from build123d import *

# Parameters (mm, degrees)
SKETCH1_W           = 57.16
SKETCH1_H           = 37.39
SKETCH1_W_2         = 40.16
SKETCH1_H_2         = 20.39
BOSS_EXTRUDE1_DEPTH = 5
SKETCH2_W           = 57.16
SKETCH2_H           = 37.39
SKETCH2_W_2         = 40.16
SKETCH2_H_2         = 20.39
BOSS_EXTRUDE2_DEPTH = 28.1
SKETCH3_W           = 48.66
SKETCH3_H           = 8.5
CUT_EXTRUDE1_DEPTH  = 28.1
CUT_EXTRUDE2_REACH  = 63.749
SKETCH5_W           = 16.39
SKETCH5_H           = 10
FILLET1_R           = 4
SKETCH6_R           = 0.95
CUT_EXTRUDE3_DEPTH  = 12
CUT_EXTRUDE4_REACH  = 63.749
SKETCH8_W           = 8.5
SKETCH8_H           = 8.5
BOSS_EXTRUDE3_DEPTH = 14.1
BOSS_EXTRUDE4_REACH = 46.226
SKETCH9_W           = 8.5
SKETCH9_H           = 24.86117923


with BuildPart() as part:
    # Sketch1 → Boss-Extrude1 (new body)
    # profile 1 of 2: a face of its own
    with BuildSketch(Plane(origin=(0, 0, 0), x_dir=(1, 0, 0), z_dir=(0, 1, 0))):
        Rectangle(SKETCH1_W, SKETCH1_H)
        Rectangle(SKETCH1_W_2, SKETCH1_H_2, mode=Mode.SUBTRACT)
    # profile 2 of 2: a face of its own
    with BuildSketch(Plane(origin=(0, 0, 0), x_dir=(1, 0, 0), z_dir=(0, 1, 0))):
        Rectangle(SKETCH1_W_2, SKETCH1_H_2)
    extrude(amount=BOSS_EXTRUDE1_DEPTH)

    # Sketch2 → Boss-Extrude2 (add)
    with BuildSketch(Plane(origin=(0, 5, 0), x_dir=(1, 0, 0), z_dir=(0, 1, 0))):
        Rectangle(SKETCH2_W, SKETCH2_H)
        Rectangle(SKETCH2_W_2, SKETCH2_H_2, mode=Mode.SUBTRACT)
    extrude(amount=BOSS_EXTRUDE2_DEPTH)

    # Sketch3 → Cut-Extrude1 (cut)
    with BuildSketch(Plane(origin=(0, 33.1, 0), x_dir=(1, 0, 0), z_dir=(0, 1, 0))):
        with Locations((-4.25, -14.445)):
            Rectangle(SKETCH3_W, SKETCH3_H)
    extrude(amount=-CUT_EXTRUDE1_DEPTH, mode=Mode.SUBTRACT)

    # Sketch5 → Cut-Extrude2 (cut, up to next)
    with BuildSketch(Plane(origin=(-20.08, 0, 0), x_dir=(0, 0, -1), z_dir=(1, 0, 0)), mode=Mode.PRIVATE) as cut_extrude2_sk1:
        with Locations((-2, 10)):
            Rectangle(SKETCH5_W, SKETCH5_H)
    cut_extrude2_tool1 = extrude(cut_extrude2_sk1.sketch, amount=-CUT_EXTRUDE2_REACH, mode=Mode.PRIVATE) & part.part
    add(cut_extrude2_tool1.solids().sort_by_distance((-20.08, 10, 2))[0], mode=Mode.SUBTRACT)

    # Fillet1
    fillet1_edges = [part.edges().sort_by_distance(p)[0] for p in [
        (-24.33, 15, 10.195),
    ]]
    fillet(fillet1_edges, radius=FILLET1_R)

    # Sketch6 → Cut-Extrude3 (cut)
    with BuildSketch(Plane(origin=(0, 33.1, 0), x_dir=(1, 0, 0), z_dir=(0, 1, 0))):
        with Locations(Location((-24.35, -4.95, 0), (0, 0, 270))):
            Circle(SKETCH6_R)
        with Locations(Location((-24.35, 4.95, 0), (0, 0, 90))):
            Circle(SKETCH6_R)
        with Locations(Location((24.35, 4.95, 0), (0, 0, 270))):
            Circle(SKETCH6_R)
        with Locations(Location((24.35, -4.95, 0), (0, 0, 90))):
            Circle(SKETCH6_R)
    extrude(amount=-CUT_EXTRUDE3_DEPTH, mode=Mode.SUBTRACT)

    # Sketch7 → Cut-Extrude4 (cut, up to next)
    with BuildSketch(Plane.ZY.offset(-20.08), mode=Mode.PRIVATE) as cut_extrude4_sk1:
        with BuildLine():
            Line((10.195, 33.1), (10.195, 19))
            ThreePointArc((10.195, 19), (9.023427125, 16.171572875), (6.195, 15))
            Line((6.195, 15), (-6.195, 15))
            Line((-6.195, 15), (-6.195, 5))
            Line((-6.195, 5), (18.695, 5))
            Line((18.695, 5), (18.695, 33.1))
            Line((18.695, 33.1), (10.195, 33.1))
        make_face()
    cut_extrude4_tool1 = extrude(cut_extrude4_sk1.sketch, amount=-CUT_EXTRUDE4_REACH, mode=Mode.PRIVATE) & part.part
    add(cut_extrude4_tool1.solids().sort_by_distance((20.08, 15.371532, 9.379812))[0], mode=Mode.SUBTRACT)

    # Sketch8 → Boss-Extrude3 (add)
    with BuildSketch(Plane(origin=(0, 33.1, 0), x_dir=(1, 0, 0), z_dir=(0, 1, 0))):
        with Locations((-24.33, -14.445)):
            Rectangle(SKETCH8_W, SKETCH8_H)
    extrude(amount=-BOSS_EXTRUDE3_DEPTH)

    # Sketch9 → Boss-Extrude4 (add, up to next)
    with BuildSketch(Plane(origin=(0, 5, 0), x_dir=(1, 0, 0), z_dir=(0, 1, 0)), mode=Mode.PRIVATE) as boss_extrude4_sk1:
        with Locations((-24.33, -6.235589615)):
            Rectangle(SKETCH9_W, SKETCH9_H)
    boss_extrude4_tool1 = extrude(boss_extrude4_sk1.sketch, amount=BOSS_EXTRUDE4_REACH, mode=Mode.PRIVATE) - part.part
    add(boss_extrude4_tool1.solids().sort_by_distance((-24.33, 5, 6.23559))[0])


solid = part.part
For this review, take the finished solid that the model builds, in its own axes (mm). A direction names the side the tool comes from. Round coordinates to 2 decimals unless told otherwise and drop trailing zeros. Loops run counter-clockwise (first coordinate to the right, second up) from the corner with the lowest first, then second, coordinate; pieces in that order, holes last. Notation, with made-up numbers: (-27.5, 22.25) - (12.5, 22.25) arc R31 cw to (12.5, 52.25) - close; hole circle Ø3 at (86, -11.75). An arc over 180 degrees is marked (long way). One line per item, written item: value. Start each with the question number.
Item 1: Clearance check with flat-ended pins moving along their axes: pin 1 Ø8.5 at (x, y) = (6.5, 21.5) entering from +Z (3 decimals); pin 2 Ø7 at (x, y) = (23, 29) entering from +Z (3 decimals); pin 3 Ø8.5 at (x, z) = (-11, 6.5) entering from +Y. State where each tip first meets the part, or that it passes through.
Item 2: For faces 1 (the flat face through (-20.08, 19, 4)), 2 (the flat face through (24, 26, 10.195)), 3 (the flat face through (24, 10, -6.195)), 4 (the flat face through (-24, 21.1, 5)), list the 3-axis set-ups (+Z, -Z, +X, -X, +Y, -Y) from which the entire face can be reached by the end or side of a thin tool; tool diameter is ignored.
Item 3: For L1, parallel to X at y = 26.25, z = -4.95; L2, parallel to X at y = 16.5, z = 7.5; L3, parallel to Y at x = 14.5, z = 16, list the stretches that pass through material, from the lowest coordinate up.
Item 4: The part is to be moulded in two halves that separate along Y. For faces 5 (the flat face through (24, 21.1, 5)), 6 (the cylindrical face through (24.27, 16.2, 9.05)), 7 (the flat face through (0, 19, -10.195)), say which applies: +Y half, -Y half, draft (parallel to the pull), parting line (faces both ways), or undercut.
Item 5: Take a section at B-B (z = 5). Give the boundary of the cut face in (x, y).
Item 6: Take a section at A-A (y = 26.5). Give the boundary of the cut face in (x, z) (3 decimals), plus the area to 3 significant figures.
Item 7: Take a section at D-D (z = 15.5). Give the boundary of the cut face in (x, y), plus the area to 3 significant figures.
Item 8: Take a section at C-C (x = -15.5). Give the boundary of the cut face in (y, z) (3 decimals).
Answer below:
1. pin 1: stops at z = -10.195
1. pin 2: stops at z = 10.195
1. pin 3: stops at y = 5
2. face 1: +Z, +Y
2. face 2: +Z, +X, +Y
2. face 3: +Z, +X
2. face 4: +Y
3. L1: x = -28.58 to -25.3, -23.4 to -20.08, 20.08 to 23.4, 25.3 to 28.58
3. L2: x = -28.58 to -20.08, 20.08 to 28.58
3. L3: y = 0 to 5
4. face 5: +Y half
4. face 6: undercut
4. face 7: draft
5. outline: (-28.58, 0) - (28.58, 0) - (28.58, 5) - (-20.08, 5) - (-20.08, 33.1) - (-23.4, 33.1) - (-23.4, 21.1) - (-25.3, 21.1) - (-25.3, 33.1) - (-28.58, 33.1) - close; (20.08, 15) - (28.58, 15) - (28.58, 33.1) - (25.3, 33.1) - (25.3, 21.1) - (23.4, 21.1) - (23.4, 33.1) - (20.08, 33.1) - close
6. outline: (-28.58, -18.695) - (28.58, -18.695) - (28.58, 10.195) - (20.08, 10.195) - (20.08, -10.195) - (-20.08, -10.195) - (-20.08, 18.695) - (-28.58, 18.695) - close; hole circle Ø1.9 at (-24.35, -4.95); hole circle Ø1.9 at (-24.35, 4.95); hole circle Ø1.9 at (24.35, -4.95); hole circle Ø1.9 at (24.35, 4.95)
6. area: 893 mm2
7. outline: (-28.58, 0) - (28.58, 0) - (28.58, 5) - (-20.08, 5) - (-20.08, 33.1) - (-28.58, 33.1) - close
7. area: 525 mm2
8. outline: (0, -18.695) - (33.1, -18.695) - (33.1, -10.195) - (5, -10.195) - (5, 18.695) - (0, 18.695) - close
